For this review, take the finished solid that the model builds, in its own axes (mm). Round coordinates to 2 decimals unless told otherwise and drop trailing zeros. Write each loop counter-clockwise with the first axis right and the second up, starting at its lowest first coordinate (ties: lowest second). Pieces come first, ordered by that corner, then holes. Notation, with made-up numbers: M 73,43 L 89,43 A15 cw 89,69 Z; hole C 27.5,80.5 d4. An arc over 180 degrees is marked long. One line per question, with ' | ' between items.
```python
from build123d import *

# Parameters (mm, degrees)
SKETCH1_W          = 62
SKETCH1_H          = 12.5
SKETCH2_R          = 8.5
CUT_EXTRUDE1_DEPTH = 63
CHAMFER2_SIZE      = 2


with BuildPart() as part:
    # Sketch1 → Revolve1 (revolve)
    with BuildSketch(Plane.XY):
        with Locations((0, 6.25)):
            Rectangle(SKETCH1_W, SKETCH1_H)
    revolve(axis=Axis((31, 0, 0), (-1, 0, 0)))

    # Sketch2 → Cut-Extrude1 (cut, through all)
    with BuildSketch(Plane(origin=(31, 0, 0), x_dir=(0, 0, -1), z_dir=(1, 0, 0))):
        Circle(SKETCH2_R)
    extrude(amount=-CUT_EXTRUDE1_DEPTH, mode=Mode.SUBTRACT)

    # Chamfer2
    chamfer2_edges = [part.edges().sort_by_distance(p)[0] for p in [
        (31, -12.5, 0),
        (-31, -12.5, 0),
    ]]
    chamfer(chamfer2_edges, length=CHAMFER2_SIZE)


solid = part.part
```
Item 1: Take a section at A-A (z = 0). Write out the cut boundary in (x, y), then the cut area to 3 significant figures.
Results:
outline: M -31,-10.5 L -29,-12.5 L 29,-12.5 L 31,-10.5 L 31,-8.5 L -31,-8.5 Z; M -31,8.5 L 31,8.5 L 31,10.5 L 29,12.5 L -29,12.5 L -31,10.5 Z | area: 488 mm2
Item 2: To check wall thickness, follow line 1 along Y through (x, z) = (0, 0); line 2 along Z through (x, y) = (18, 5.5); line 3 along Y through (x, z) = (-21, -1). State the ranges of each line that lie inside material, in increasing order. Write a range as from..to.
Results:
line 1: -12.5..-8.5, 8.5..12.5 | line 2: -11.22..-6.48, 6.48..11.22 | line 3: -12.46..-8.44, 8.44..12.46
Item 3: Mouldability with a two-part tool opening along Z and no side actions: class faces 1 (the face through (0.434, 7.167, -4.57)), 2 (the face through (0.406, 11.923, -3.755)), 3 (the face through (31, -9, 0)) as +Z half, -Z half, draft (parallel to the pull), parting line (faces both ways), or undercut.
Results:
face 1: undercut | face 2: parting line | face 3: draft
Item 4: Insertion check: pin 1 Ø5 at (x, y) = (6.5, -8.5) entering from -Z; pin 2 Ø13.5 at (y, z) = (0, 0) entering from +X. Each pin has a flat end and moves straight along its axis. Give the tip position at first contact, or say it passes through.
Results:
pin 1: z = -10.97 | pin 2: through
Item 5: Take a section at C-C (x = 9.5). Write out the cut boundary in (y, z).
Results:
outline: C 0,0 d25; hole C 0,0 d17
